Source: CAD feature listing. Evaluate the final solid. Frame: model axes, mm. A direction names the side the tool comes from. Give positions to 0.01 mm unless a question says otherwise; leave off trailing zeros. Loops run counter-clockwise (first coordinate to the right, second up) from the corner with the lowest first, then second, coordinate; pieces in that order, holes last. Notation, with made-up numbers: M -2.5,61 L 44.5,61 A5 cw 44.5,66 Z; hole C 9,60.5 d4. An arc over 180 degrees is marked long. Answer in a Markdown table with one row per item.
```python
from build123d import *
from OCP.BRepFilletAPI import BRepFilletAPI_MakeChamfer

# Parameters (mm, degrees)
ESTRUSIONE_ESTRUSIONE1_DEPTH = 2
ESTRUSIONE_ESTRUSIONE2_DEPTH = 1
SCHIZZO3_R                   = 4
SCHIZZO3_R_2                 = 1.75
ESTRUSIONE_ESTRUSIONE3_DEPTH = 12.5
TAGLIO_ESTRUSIONE1_START     = -13
SCHIZZO4_R                   = 1.75
TAGLIO_ESTRUSIONE1_DEPTH     = 13
SCHIZZO5_W                   = 24
SCHIZZO5_H                   = 13
TAGLIO_ESTRUSIONE2_DEPTH     = 13
SCHIZZO6_W                   = 35
SCHIZZO6_H                   = 23
TAGLIO_ESTRUSIONE3_DEPTH     = 1
RACCORDO1_R                  = 2
RACCORDO2_R                  = 2
SMUSSO1_SIZE                 = 1.5
SMUSSO2_SIZE                 = 1.5
SMUSSO2_SIZE2                = 1.787630389
SCHIZZO7_R                   = 3.25
SCHIZZO7_R_2                 = 1.75
ESTRUSIONE_ESTRUSIONE4_DEPTH = 7
TAGLIO_ESTRUSIONE4_START     = -10
SCHIZZO8_R                   = 1.75
TAGLIO_ESTRUSIONE4_DEPTH     = 10


with BuildPart() as part:
    # Schizzo1 → Estrusione-Estrusione1 (new body)
    with BuildSketch(Plane.XY):
        with BuildLine():
            Line((-34, -24), (34, -24))
            ThreePointArc((34, -24), (37.535533906, -22.535533906), (39, -19))
            Line((39, -19), (39, 19))
            ThreePointArc((39, 19), (37.535533906, 22.535533906), (34, 24))
            Line((34, 24), (-34, 24))
            ThreePointArc((-34, 24), (-37.535533906, 22.535533906), (-39, 19))
            Line((-39, 19), (-39, -19))
            ThreePointArc((-39, -19), (-37.535533906, -22.535533906), (-34, -24))
        make_face()
    extrude(amount=ESTRUSIONE_ESTRUSIONE1_DEPTH)

    # Schizzo2 → Estrusione-Estrusione2 (add)
    with BuildSketch(Plane(origin=(0, 0, 0), x_dir=(-1, 0, 0), z_dir=(0, 0, -1))):
        with BuildLine():
            Line((-36.5, -18), (-36.5, 18))
            ThreePointArc((-36.5, 18), (-35.474873734, 20.474873734), (-33, 21.5))
            Line((-33, 21.5), (33, 21.5))
            ThreePointArc((33, 21.5), (35.474873734, 20.474873734), (36.5, 18))
            Line((36.5, 18), (36.5, -18))
            ThreePointArc((36.5, -18), (35.474873734, -20.474873734), (33, -21.5))
            Line((33, -21.5), (-33, -21.5))
            ThreePointArc((-33, -21.5), (-35.474873734, -20.474873734), (-36.5, -18))
        make_face()
    extrude(amount=ESTRUSIONE_ESTRUSIONE2_DEPTH)

    # Schizzo3 → Estrusione-Estrusione3 (add)
    # profile 1 of 3: a face of its own
    with BuildSketch(Plane(origin=(0, 0, -1), x_dir=(-1, 0, 0), z_dir=(0, 0, -1))):
        with Locations((-31, 16)):
            Circle(SCHIZZO3_R)
        with Locations((-31, 16)):
            Circle(SCHIZZO3_R_2, mode=Mode.SUBTRACT)
    # profile 2 of 3: a face of its own
    with BuildSketch(Plane(origin=(0, 0, -1), x_dir=(-1, 0, 0), z_dir=(0, 0, -1))):
        with Locations((-31, -16)):
            Circle(SCHIZZO3_R)
        with Locations((-31, -16)):
            Circle(SCHIZZO3_R_2, mode=Mode.SUBTRACT)
    # profile 3 of 3: a face of its own
    with BuildSketch(Plane(origin=(0, 0, -1), x_dir=(-1, 0, 0), z_dir=(0, 0, -1))):
        with Locations((31, 16)):
            Circle(SCHIZZO3_R)
        with Locations((31, 16)):
            Circle(SCHIZZO3_R_2, mode=Mode.SUBTRACT)
    extrude(amount=ESTRUSIONE_ESTRUSIONE3_DEPTH)

    # Schizzo4 → Taglio-Estrusione1 (cut)
    with BuildSketch(Plane(origin=(0, 0, -1), x_dir=(-1, 0, 0), z_dir=(0, 0, -1)).offset(TAGLIO_ESTRUSIONE1_START)):
        with Locations((-31, -16)):
            Circle(SCHIZZO4_R)
        with Locations((-31, 16)):
            Circle(SCHIZZO4_R)
        with Locations((31, 16)):
            Circle(SCHIZZO4_R)
        with Locations((31, -16)):
            Circle(SCHIZZO4_R)
    extrude(amount=TAGLIO_ESTRUSIONE1_DEPTH, mode=Mode.SUBTRACT)

    # Schizzo5 → Taglio-Estrusione2 (cut)
    with BuildSketch(Plane(origin=(0, 0, -1), x_dir=(-1, 0, 0), z_dir=(0, 0, -1))):
        with Locations((15.8, -0.5)):
            Rectangle(SCHIZZO5_W, SCHIZZO5_H)
    extrude(amount=-TAGLIO_ESTRUSIONE2_DEPTH, mode=Mode.SUBTRACT)

    # Schizzo6 → Taglio-Estrusione3 (cut)
    with BuildSketch(Plane(origin=(0, 0, -1), x_dir=(-1, 0, 0), z_dir=(0, 0, -1))):
        with Locations((15.8, -0.5)):
            Rectangle(SCHIZZO6_W, SCHIZZO6_H)
    extrude(amount=-TAGLIO_ESTRUSIONE3_DEPTH, mode=Mode.SUBTRACT)

    # Raccordo1
    raccordo1_edges = [part.edges().sort_by_distance(p)[0] for p in [
        (-37.535533906, 22.535533906, 2),
        (0, 24, 2),
        (37.535533906, 22.535533906, 2),
        (39, 0, 2),
        (37.535533906, -22.535533906, 2),
        (0, -24, 2),
        (-37.535533906, -22.535533906, 2),
        (-39, 0, 2),
    ]]
    fillet(raccordo1_edges, radius=RACCORDO1_R - 0.0001)  # a hair under: the kernel refuses the full size

    # Raccordo2
    raccordo2_edges = [part.edges().sort_by_distance(p)[0] for p in [
        (-3.8, -7, 1),
        (-3.8, 6, 1),
        (-27.8, 6, 1),
        (-27.8, -7, 1),
    ]]
    fillet(raccordo2_edges, radius=RACCORDO2_R)

    # Smusso1
    smusso1_edges = [part.edges().sort_by_distance(p)[0] for p in [
        (-27.8, -0.5, 2),
        (-15.8, -7, 2),
        (-3.8, -0.5, 2),
        (-15.8, 6, 2),
        (-27.214213562, -6.414213562, 2),
        (-4.385786438, -6.414213562, 2),
        (-4.385786438, 5.414213562, 2),
        (-27.214213562, 5.414213562, 2),
    ]]
    chamfer(smusso1_edges, length=SMUSSO1_SIZE)

    # Smusso2: one chamfer whose edges measure the first distance from different faces: ONE call of the kernel's chamfer builder (chamfer() names one face for all edges)
    smusso2_edges_1 = [part.edges().sort_by_distance(p)[0] for p in [
        (-29.25, -16, 2),
    ]]
    smusso2_side_1 = [part.faces().sort_by_distance(p)[0] for p in [
        (-29.25, -16, 0.5),
    ]]
    smusso2_edges_2 = [part.edges().sort_by_distance(p)[0] for p in [
        (-29.25, 16, 2),
    ]]
    smusso2_side_2 = [part.faces().sort_by_distance(p)[0] for p in [
        (-29.25, 16, -5.75),
    ]]
    smusso2_edges_3 = [part.edges().sort_by_distance(p)[0] for p in [
        (32.75, 16, 2),
    ]]
    smusso2_side_3 = [part.faces().sort_by_distance(p)[0] for p in [
        (32.75, 16, -5.75),
    ]]
    smusso2_edges_4 = [part.edges().sort_by_distance(p)[0] for p in [
        (32.75, -16, 2),
    ]]
    smusso2_side_4 = [part.faces().sort_by_distance(p)[0] for p in [
        (32.75, -16, -5.75),
    ]]
    smusso2 = BRepFilletAPI_MakeChamfer(part.part.solid().wrapped)
    for e in smusso2_edges_1:
        smusso2.Add(SMUSSO2_SIZE, SMUSSO2_SIZE2, e.wrapped, smusso2_side_1[0].wrapped)  # the first distance lies on this face
    for e in smusso2_edges_2:
        smusso2.Add(SMUSSO2_SIZE, SMUSSO2_SIZE2, e.wrapped, smusso2_side_2[0].wrapped)  # the first distance lies on this face
    for e in smusso2_edges_3:
        smusso2.Add(SMUSSO2_SIZE, SMUSSO2_SIZE2, e.wrapped, smusso2_side_3[0].wrapped)  # the first distance lies on this face
    for e in smusso2_edges_4:
        smusso2.Add(SMUSSO2_SIZE, SMUSSO2_SIZE2, e.wrapped, smusso2_side_4[0].wrapped)  # the first distance lies on this face
    add(Compound.cast(smusso2.Shape()), mode=Mode.REPLACE)

    # Schizzo7 → Estrusione-Estrusione4 (add)
    # profile 1 of 3: a face of its own
    with BuildSketch(Plane(origin=(0, 0, -1), x_dir=(-1, 0, 0), z_dir=(0, 0, -1))):
        with Locations((-14.5, 12)):
            Circle(SCHIZZO7_R)
        with Locations((-14.5, 12)):
            Circle(SCHIZZO7_R_2, mode=Mode.SUBTRACT)
    # profile 2 of 3: a face of its own
    with BuildSketch(Plane(origin=(0, 0, -1), x_dir=(-1, 0, 0), z_dir=(0, 0, -1))):
        with Locations((-14.5, 0)):
            Circle(SCHIZZO7_R)
        with Locations((-14.5, 0)):
            Circle(SCHIZZO7_R_2, mode=Mode.SUBTRACT)
    # profile 3 of 3: a face of its own
    with BuildSketch(Plane(origin=(0, 0, -1), x_dir=(-1, 0, 0), z_dir=(0, 0, -1))):
        with Locations((-14.5, -12)):
            Circle(SCHIZZO7_R)
        with Locations((-14.5, -12)):
            Circle(SCHIZZO7_R_2, mode=Mode.SUBTRACT)
    extrude(amount=ESTRUSIONE_ESTRUSIONE4_DEPTH)

    # Schizzo8 → Taglio-Estrusione4 (cut)
    with BuildSketch(Plane(origin=(0, 0, -1), x_dir=(-1, 0, 0), z_dir=(0, 0, -1)).offset(TAGLIO_ESTRUSIONE4_START)):
        with Locations((-14.5, 12)):
            Circle(SCHIZZO8_R)
        with Locations((-14.5, 0)):
            Circle(SCHIZZO8_R)
        with Locations((-14.5, -12)):
            Circle(SCHIZZO8_R)
    extrude(amount=TAGLIO_ESTRUSIONE4_DEPTH, mode=Mode.SUBTRACT)


solid = part.part
```
1) Pin query (flat end, axial travel): pin 1 Ø2 at (x, y) = (15, 1) entering from -Z; pin 2 Ø5 at (x, y) = (-5, 2.5) entering from -Z; pin 3 Ø0.8 at (y, z) = (1.5, -0.5) entering from +X. Return the tip coordinate at first contact, or that it passes through.
Reply:
| item | result |
|---|---|
| pin 1 | stops at z = -8 |
| pin 2 | stops at z = 0 |
| pin 3 | stops at x = 36.5 |
2) Section A-A, the plane z = -11.25. Return loops of the section in (x, y), then the cut area to 3 significant figures.
Reply:
| item | result |
|---|---|
| outline | C -31,16 d8; C 31,-16 d8; C 31,16 d8; hole C -31,16 d3.5; hole C 31,-16 d3.5; hole C 31,16 d3.5 |
| area | 122 mm² |
3) Section B-B, the plane y = 0. Count the separate pieces of the cut face and the enclosed holes in it, then the cut area to 3 significant figures.
Reply:
| item | result |
|---|---|
| separate pieces | 3 |
| enclosed holes | 0 |
| area | 153 mm² |
4) Pull-direction query (X, two-part tool) for faces 1 (the cylindrical face through (-35.45, 20.5, -0.49)), 2 (the cylindrical face through (-27.23, -6.4, 0.25)), 3 (the cylindrical face through (35.5, 20.45, -0.49)); classes: released by +X, released by -X, zero draft, split by the parting line, or undercut.
Reply:
| item | result |
|---|---|
| face 1 | released by -X |
| face 2 | undercut |
| face 3 | released by +X |
5) Set-up query: faces 4 (the conical face through (-27.639, -6.799, 1.073)), 5 (the cylindrical face through (-38.4, -0.27, 1.43)), 6 (the cylindrical face through (17.747, 0.143, -4.451)), 7 (the cylindrical face through (-27.2, 5.43, 0.25)). Return all of +Z, -Z, +X, -X, +Y, -Y with unobstructed straight access to the full face (end or side cutting, diameter ignored); none if empty.
Reply:
| item | result |
|---|---|
| face 4 | +Z |
| face 5 | +Z, -X, +Y, -Y |
| face 6 | -Z |
| face 7 | +Z, -Z |
6) Material intervals for L1, parallel to Y at x = 14.5, z = -4.75; L2, parallel to X at y = -16, z = 0.15; L3, parallel to Y at x = 14.5, z = -0.25, sorted ascending.
Reply:
| item | result |
|---|---|
| L1 | y = -15.25 to -13.75, -10.25 to -8.75, -3.25 to -1.75, 1.75 to 3.25, 8.75 to 10.25, 13.75 to 15.25 |
| L2 | x = -38.99 to -32.75, -29.25 to 29.25, 32.75 to 38.99 |
| L3 | y = -21.5 to -13.75, -10.25 to -1.75, 1.75 to 10.25, 13.75 to 21.5 |
